```python
from build123d import *

# Parameters (mm, degrees)
F0_W     = 50.8
F0_H     = 25.4
F1_DEPTH = 177.8
F3_W     = 47.625
F3_H     = 22.225
F4_DEPTH = 203.2
F2_R     = 2.5527
F5_DEPTH = 76.2
F6_R     = 2.5527
F7_DEPTH = 50.8
F6_R_2   = 14.2875
F8_DEPTH = 50.8


# Not quite as in the source:
# - a feature names something its author has since deleted; it is built from what else it names


with BuildPart() as f1:
    # F0 (on Front) → F1 (new body)
    with BuildSketch(Plane.XZ):
        Rectangle(F0_W, F0_H)
    extrude(amount=F1_DEPTH)

    # F3 (on face) → F4 (cut)
    with BuildSketch(Plane.XZ.offset(177.8)):
        Rectangle(F3_W, F3_H)
    extrude(amount=-F4_DEPTH, mode=Mode.SUBTRACT)

    # F2 (on face) → F5 (cut)
    with BuildSketch(Plane.YZ.offset(25.4)):
        with Locations((-165.1, 0)):
            Circle(F2_R)
        with Locations((-139.7, 0)):
            Circle(F2_R)
        with Locations((-114.3, 0)):
            Circle(F2_R)
        with Locations((-88.9, 0)):
            Circle(F2_R)
        with Locations((-63.5, 0)):
            Circle(F2_R)
        with Locations((-38.1, 0)):
            Circle(F2_R)
        with Locations((-12.7, 0)):
            Circle(F2_R)
        with Locations((12.7, 0)):
            Circle(F2_R)
    extrude(amount=-F5_DEPTH, mode=Mode.SUBTRACT)

    # F6 (on face) → F7 (cut)
    with BuildSketch(Plane(origin=(0, 0, -12.7), x_dir=(1, 0, 0), z_dir=(0, 0, -1))):
        with Locations((-12.7, 165.1)):
            Circle(F6_R)
        with Locations((-12.7, 139.7)):
            Circle(F6_R)
        with Locations((-12.7, 114.3)):
            Circle(F6_R)
        with Locations((-12.7, 88.9)):
            Circle(F6_R)
        with Locations((-12.7, 63.5)):
            Circle(F6_R)
        with Locations((12.7, 63.5)):
            Circle(F6_R)
        with Locations((12.7, 88.9)):
            Circle(F6_R)
        with Locations((12.7, 114.3)):
            Circle(F6_R)
        with Locations((12.7, 139.7)):
            Circle(F6_R)
        with Locations((12.7, 165.1)):
            Circle(F6_R)
    extrude(amount=-F7_DEPTH, mode=Mode.SUBTRACT)

    # F6 (on face) → F8 (cut)
    with BuildSketch(Plane(origin=(0, 0, -12.7), x_dir=(1, 0, 0), z_dir=(0, 0, -1))):
        with Locations((0, 25.4)):
            Circle(F6_R_2)
    extrude(amount=-F8_DEPTH, mode=Mode.SUBTRACT)


solid = f1.part
```
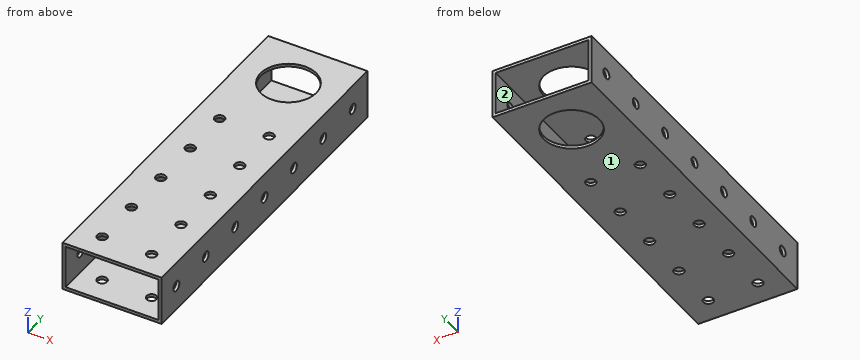
Check sheet for the modelled part. Datum: model origin and axes. Units: mm. Face numbers are marked on the shaded views. A direction names the side the tool comes from. Give positions to 0.01 mm unless a question says otherwise; leave off trailing zeros. Loops run counter-clockwise (first coordinate to the right, second up) from the corner with the lowest first, then second, coordinate; pieces in that order, holes last. Notation, with made-up numbers: (5.25, -28) - (32.25, -28) arc R17 cw to (32.25, -15) - close; hole circle Ø11 at (38.25, -2.75). An arc over 180 degrees is marked (long way). One line per question, with ' | ' between items. Start each with the question number.
1. Material ranges on line 1 along X through (y, z) = (-88.9, -12.25); line 2 along X through (y, z) = (-26, 1); line 3 along Z through (x, y) = (-18, -78.5), recorded low to high. Write a range as [from, to].
2. Cross-section at A-A, the plane y = -63.5. Give the number of separate pieces and of enclosed holes in the cut face, plus the area to 3 significant figures.
3. Cross-section at C-C, the plane z = 9. Enter the section's corners in (x, y).
4. Set-up check for the marked faces 1 and 2: record each of +Z, -Z, +X, -X, +Y, -Y from which the full face is reachable in a straight line by a thin tool's end or side.
5. Cross-section at D-D, the plane x = 6.5. Enter the section's corners in (y, z).
6. Cross-section at B-B, the plane x = -21.5. Enter the section's corners in (y, z), plus the area to 3 significant figures.
Check result:
1) line 1: x = [-25.4, -15.25], [-10.15, 10.15], [15.25, 25.4] | line 2: x = [-25.4, -23.81], [23.81, 25.4] | line 3: z = [-12.7, -11.11], [11.11, 12.7]
2) separate pieces: 6 | enclosed holes: 0 | area: 183 mm2
3) outline: (-25.4, -177.8) - (-23.81, -177.8) - (-23.81, 0) - (-25.4, 0) - close; (23.81, -177.8) - (25.4, -177.8) - (25.4, 0) - (23.81, 0) - close
4) face 1: -Z, +X, -X, +Y, -Y | face 2: +Y, -Y
5) outline: (-177.8, -12.7) - (-38.12, -12.7) - (-38.12, -11.11) - (-177.8, -11.11) - close; (-177.8, 11.11) - (-38.12, 11.11) - (-38.12, 12.7) - (-177.8, 12.7) - close; (-12.68, -12.7) - (0, -12.7) - (0, -11.11) - (-12.68, -11.11) - close; (-12.68, 11.11) - (0, 11.11) - (0, 12.7) - (-12.68, 12.7) - close
6) outline: (-177.8, -12.7) - (0, -12.7) - (0, -11.11) - (-177.8, -11.11) - close; (-177.8, 11.11) - (0, 11.11) - (0, 12.7) - (-177.8, 12.7) - close | area: 565 mm2
